Verification items for the finished model (mm, model axes). Face numbers are marked on the shaded views. Coordinates: 2 decimals unless noted, no trailing zeros. Order: outer loops, then holes, each group sorted by start corner. A loop starts at its lowest first (then second) coordinate and runs counter-clockwise, first axis right, second up. Notation, with made-up numbers: M -36.75,70 L 13.25,70 A14 cw 13.25,90 Z; hole C -16.75,68 d3. An arc over 180 degrees is marked long. Use one line per item in the form item = value. Start each with the question number.
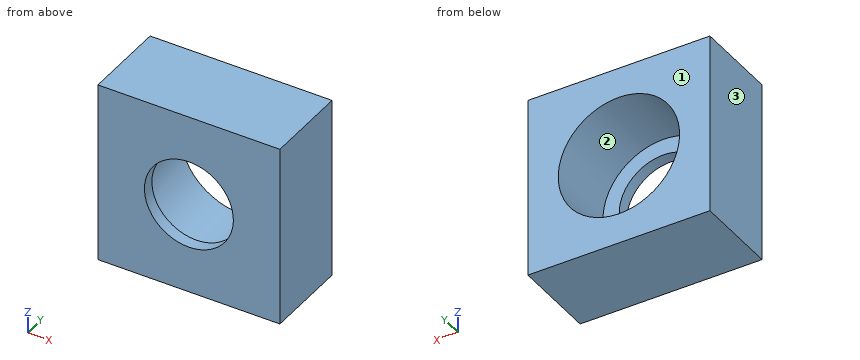
```python
from build123d import *

# Parameters (mm, degrees)
SKETCH2_W           = 45
SKETCH2_H           = 45
SKETCH2_R           = 11
BOSS_EXTRUDE1_DEPTH = 21
SKETCH3_R           = 15
CUT_EXTRUDE1_DEPTH  = 18


with BuildPart() as part:
    # Sketch2 → Boss-Extrude1 (new body)
    with BuildSketch(Plane(origin=(0, 0, 0), x_dir=(1, 0, 0), z_dir=(0, 1, 0))):
        Rectangle(SKETCH2_W, SKETCH2_H)
        with Locations(Location((0, 0, 0), (0, 0, 90))):
            Circle(SKETCH2_R, mode=Mode.SUBTRACT)
    extrude(amount=BOSS_EXTRUDE1_DEPTH)

    # Sketch3 → Cut-Extrude1 (cut)
    with BuildSketch(Plane(origin=(0, 21, 0), x_dir=(1, 0, 0), z_dir=(0, 1, 0))):
        with Locations(Location((0, 0, 0), (0, 0, 270))):
            Circle(SKETCH3_R)
    extrude(amount=-CUT_EXTRUDE1_DEPTH, mode=Mode.SUBTRACT)


solid = part.part
```
1. Material ranges on line 1 along X through (y, z) = (10.25, 0); line 2 along X through (y, z) = (1.15, 0); line 3 along Y through (x, z) = (11, -8.5), recorded low to high.
2. Depth check by flat-ended pin: P1, Ø18, axis at x = 0, z = 0, coming from the +Y side. Enter the tip coordinate at first touch or a pass-through.
3. Release check for a two-part mould opening along X. For the marked faces 1, 2 and 3 record: pulls with the +X half, pulls with the -X half, needs draft (parallel to the pull), parting line crosses it, or undercut.
4. Cross-section at D-D on x = 13. Enter the section's corners in (y, z), and give its area (3 significant figures).
5. Cross-section at B-B on x = 0. Enter the section's corners in (y, z), and give its area (3 significant figures).
6. Cross-section at A-A on z = 0. Enter the section's corners in (x, y).
7. Cross-section at C-C on y = 13.25. Enter the section's corners in (x, z).
Final values:
q1.line_1 = -22.5 to -15, 15 to 22.5
q1.line_2 = -22.5 to -11, 11 to 22.5
q1.line_3 = 0 to 3
q2.P1 = through
q3.face_1 = needs draft
q3.face_2 = undercut
q3.face_3 = pulls with the -X half
q4.outline = M 0,-22.5 L 21,-22.5 L 21,-7.48 L 3,-7.48 L 3,7.48 L 21,7.48 L 21,22.5 L 0,22.5 Z
q4.area = 676 mm2
q5.outline = M 0,-22.5 L 21,-22.5 L 21,-15 L 3,-15 L 3,-11 L 0,-11 Z; M 0,11 L 3,11 L 3,15 L 21,15 L 21,22.5 L 0,22.5 Z
q5.area = 339 mm2
q6.outline = M -22.5,0 L -11,0 L -11,3 L -15,3 L -15,21 L -22.5,21 Z; M 11,0 L 22.5,0 L 22.5,21 L 15,21 L 15,3 L 11,3 Z
q7.outline = M -22.5,-22.5 L 22.5,-22.5 L 22.5,22.5 L -22.5,22.5 Z; hole C 0,0 d30
